Geometry check sheet. Reference: the model listing, model coordinates, mm. A direction names the side the tool comes from. Give positions to 0.01 mm unless a question says otherwise; leave off trailing zeros. Loops run counter-clockwise (first coordinate to the right, second up) from the corner with the lowest first, then second, coordinate; pieces in that order, holes last. Notation, with made-up numbers: (-14, 51.5) -> (18, 51.5) arc R23 ccw to (18, 74.5) -> close; hole circle Ø6 at (1, 48.5). An arc over 180 degrees is marked (long way). Answer in a Markdown table with one row per item. Add a question column.
```python
from build123d import *

# Parameters (mm, degrees)
F0_R     = 4
F0_R_2   = 3
F1_DEPTH = 1
F0_R_3   = 1.875
F2_DEPTH = 3.7
F3_R     = 3
F3_R_2   = 1.875
F4_DEPTH = 2
F5_R     = 2


with BuildPart() as f1:
    # F0 (on Top) → F1 (new body)
    with BuildSketch(Plane.XY):
        with Locations((-0.725, 0)):
            Circle(F0_R)
        with Locations((-0.725, 0)):
            Circle(F0_R_2, mode=Mode.SUBTRACT)
    extrude(amount=F1_DEPTH)

    # F0 (on Top) → F2 (join)
    with BuildSketch(Plane.XY):
        with Locations((-0.725, 0)):
            Circle(F0_R_2)
        Circle(F0_R_3, mode=Mode.SUBTRACT)
    extrude(amount=F2_DEPTH)

    # F3 (on face) → F4 (join)
    with BuildSketch(Plane.XY.offset(3.7)):
        with Locations((-0.725, 0)):
            Circle(F3_R)
        Circle(F3_R_2, mode=Mode.SUBTRACT)
        Circle(F3_R_2)
    extrude(amount=F4_DEPTH)

    # F5
    f5_edges = [f1.edges().sort_by_distance(p)[0] for p in [
        (-3.725, 0, 5.7),
    ]]
    fillet(f5_edges, radius=F5_R)


solid = f1.part
```
1. Release check for a two-part mould opening along Y. For faces 4 (the face through (-1.873, 0.082, 1.824)), 5 (the face through (-3.722, 0.132, 2.331)), 6 (the face through (-2, 1, 0)) record: released by +Y, released by -Y, zero draft, split by the parting line, or undercut.
2. Material ranges on L1, parallel to Y at x = 0.25, z = 3.5; L2, parallel to Z at x = -1.5, y = -0.25; L3, parallel to Z at x = -3.25, y = 2.25, recorded low to high. Write a range as from..to.
3. Gauge pin test, flat end, axial feed: pin 1 Ø2 at (y, z) = (-2, 2.5) entering from +X. Record the tip position at first contact, or that the pin passes through.
4. Sectioned sample at B-B (x = -4). Enter the section's corners in (y, z).
5. Sectioned sample at A-A (z = 0.65). Enter the section's corners in (x, y) (3 decimals).
6. Access from +Z, -Z, +X, -X, +Y, -Y to the whole of each face (thin tool, end or side, straight path). Record for faces 1 (the face through (0, 0, 3.7)), 2 (the face through (1, 3, 1)), 3 (the face through (-1.592, -3.905, 0.493)).
Response:
| question | item | result |
|---|---|---|
| 1 | face 4 | undercut |
| 1 | face 5 | split by the parting line |
| 1 | face 6 | zero draft |
| 2 | L1 | y = -2.84..-1.86, 1.86..2.84 |
| 2 | L2 | z = 3.7..5.7 |
| 2 | L3 | z = 0..1 |
| 3 | pin 1 | stops at x = 2.1 |
| 4 | outline | (-2.3, 0) -> (2.3, 0) -> (2.3, 1) -> (-2.3, 1) -> close |
| 5 | outline | circle Ø8 at (-0.725, 0); hole circle Ø3.75 at (0, 0) |
| 6 | face 1 | -Z |
| 6 | face 2 | +Z |
| 6 | face 3 | +Z, -Z |
